```python
from build123d import *

# Parameters (mm, degrees)
CROQUIS1_W             = 85
CROQUIS1_H             = 100
BRIDA_BASE3_DEPTH      = 3
BRIDA_DE_ARISTA1_DEPTH = 85
CROQUIS21_R            = 2.5
CORTAR_EXTRUIR3_DEPTH  = 35
REDONDEO3_R            = 5
REDONDEO4_R            = 5
BRIDA_DE_ARISTA2_DEPTH = 85
REDONDEO5_R            = 5


# Sheet-metal steps are written as plain solids
with BuildPart() as part:
    # Croquis1 → Brida base3 (new body)
    with BuildSketch(Plane.XY):
        Rectangle(CROQUIS1_W, CROQUIS1_H)
    extrude(amount=-BRIDA_BASE3_DEPTH)

    # Brida de arista1 section (across the edge) → Brida de arista1 (add)
    with BuildSketch(Plane(origin=(-42.5, 50.828427125, -3), x_dir=(0, -0.7071067811865438, -0.7071067811865512), z_dir=(1, 0, 0))):
        with BuildLine():
            Line((-3, 0.828427125), (-3, 68.757359313))
            Line((-3, 68.757359313), (0, 68.757359313))
            Line((0, 68.757359313), (0, 0.828427125))
            ThreePointArc((0, 0.828427125), (0.152240935, 0.06306026), (0.585786438, -0.585786438))
            Line((0.585786438, -0.585786438), (-1.535533906, -2.707106781))
            ThreePointArc((-1.535533906, -2.707106781), (-2.619397663, -1.084990037), (-3, 0.828427125))
        make_face()
    extrude(amount=BRIDA_DE_ARISTA1_DEPTH)

    # Croquis21 → Cortar-Extruir3 (cut)
    with BuildSketch(Plane.XY):
        Circle(CROQUIS21_R)
        with Locations((24, 0)):
            Circle(CROQUIS21_R)
        with Locations((-24, 0)):
            Circle(CROQUIS21_R)
    extrude(amount=-CORTAR_EXTRUIR3_DEPTH, mode=Mode.SUBTRACT)

    # Redondeo3
    redondeo3_edges = [part.edges().sort_by_distance(p)[0] for p in [
        (42.5, -50, -1.5),
    ]]
    fillet(redondeo3_edges, radius=REDONDEO3_R)

    # Redondeo4
    redondeo4_edges = [part.edges().sort_by_distance(p)[0] for p in [
        (-42.5, -50, -1.5),
    ]]
    fillet(redondeo4_edges, radius=REDONDEO4_R)

    # Brida de arista2 section (across the edge) → Brida de arista2 (add)
    with BuildSketch(Plane(origin=(-42.5, 100.033008589, -52.204581464), x_dir=(0, -1, 0), z_dir=(1, 0, 0))):
        with BuildLine():
            Line((-3, 0.828427125), (-3, 78.757359313))
            Line((-3, 78.757359313), (0, 78.757359313))
            Line((0, 78.757359313), (0, 0.828427125))
            ThreePointArc((0, 0.828427125), (0.152240935, 0.06306026), (0.585786438, -0.585786438))
            Line((0.585786438, -0.585786438), (-1.535533906, -2.707106781))
            ThreePointArc((-1.535533906, -2.707106781), (-2.619397663, -1.084990037), (-3, 0.828427125))
        make_face()
    extrude(amount=BRIDA_DE_ARISTA2_DEPTH)

    # Redondeo5
    redondeo5_edges = [part.edges().sort_by_distance(p)[0] for p in [
        (-42.5, 101.533008589, -130.961940777),
        (42.5, 101.533008589, -130.961940777),
    ]]
    fillet(redondeo5_edges, radius=REDONDEO5_R)


solid = part.part
```
Check sheet for the modelled part. Datum: model origin and axes. Units: mm. A direction names the side the tool comes from. Coordinates: 2 decimals unless noted, no trailing zeros. Write each loop counter-clockwise with the first axis right and the second up, starting at its lowest first coordinate (ties: lowest second). Pieces come first, ordered by that corner, then holes. Notation, with made-up numbers: M 27,28.5 L 44,28.5 A22 ccw 44,62.5 Z; hole C 87.5,-37 d6. An arc over 180 degrees is marked long. Write item = value, one per line. Start each with the question number.
1. Sectioned sample at D-D (z = -38.5). Record the cut outline in (x, y), then the cut area to 3 significant figures.
2. Sectioned sample at A-A (y = 0). Record the cut outline in (x, z).
3. Tool access check on faces 4 (the cylindrical face through (-0.59, 102.64, -51.09)), 5 (the flat face through (-1, 100.033, -93)). Record the directions out of +Z, -Z, +X, -X, +Y, -Y that give a thin tool (end or side, any length) a straight path to the whole face; none if there is none.
4. Sectioned sample at B-B (x = 0). Record the cut outline in (y, z).
5. Sectioned sample at C-C (x = 32). Record the cut outline in (y, z).
6. Mould release check, pull along Y, two halves, no side actions. Record for faces 1 (the flat face through (-0.59, 75.77, -27.94)), 2 (the cylindrical face through (-0.54, -2.44, -1.48)), 3 (the flat face through (-1, 103.033, -91)): pulls with the +Y half, pulls with the -Y half, needs draft (parallel to the pull), parting line crosses it, or undercut.
7. Thickness scan on probe 1 along Z at (x, y) = (-22, 41.5); probe 2 along Y at (x, z) = (24, -1); probe 3 along Y at (x, z) = (0, -2.3). Record the ranges inside material, lowest first.
8. Go/stop test with flat-tipped pins: pin 1 (6.5 mm diameter, centred on x = 24, y = 0, fed in from -Z); pin 2 (6 mm diameter, centred on x = -10, z = -90.5, fed in from -Y); pin 3 (1.5 mm diameter, centred on x = 22.5, y = 80.5, fed in from +Z). Record where each tip stops, or that it passes through.
The answers:
q1.outline = M -42.5,86.33 L 42.5,86.33 L 42.5,90.57 L -42.5,90.57 Z
q1.area = 361 mm²
q2.outline = M -42.5,-3 L -26.5,-3 L -26.5,0 L -42.5,0 Z; M -21.5,-3 L -2.5,-3 L -2.5,0 L -21.5,0 Z; M 2.5,-3 L 21.5,-3 L 21.5,0 L 2.5,0 Z; M 26.5,-3 L 42.5,-3 L 42.5,0 L 26.5,0 Z
q3.face_4 = +Z, +X, -X, +Y
q3.face_5 = -Z, +X, -X, -Y
q4.outline = M -50,-3 L -2.5,-3 L -2.5,0 L -50,0 Z; M 2.5,-3 L 50,-3 A2 cw 51.41,-3.59 L 99.45,-51.62 A2 cw 100.03,-53.03 L 100.03,-130.96 L 103.03,-130.96 L 103.03,-53.03 A5 ccw 101.57,-49.5 L 53.54,-1.46 A5 ccw 50,0 L 2.5,0 Z
q5.outline = M -50,-3 L 50,-3 A2 cw 51.41,-3.59 L 99.45,-51.62 A2 cw 100.03,-53.03 L 100.03,-130.96 L 103.03,-130.96 L 103.03,-53.03 A5 ccw 101.57,-49.5 L 53.54,-1.46 A5 ccw 50,0 L -50,0 Z
q6.face_1 = pulls with the -Y half
q6.face_2 = undercut
q6.face_3 = pulls with the +Y half
q7.probe_1 = -3 to 0
q7.probe_2 = -50 to -2.5, 2.5 to 53
q7.probe_3 = -50 to -2.5, 2.5 to 54.37
q8.pin_1 = -3
q8.pin_2 = 100.03
q8.pin_3 = -27.68
